Geometry check sheet. Reference: the model listing, model coordinates, mm. A direction names the side the tool comes from. Round coordinates to 2 decimals unless told otherwise and drop trailing zeros. Loops run counter-clockwise (first coordinate to the right, second up) from the corner with the lowest first, then second, coordinate; pieces in that order, holes last. Notation, with made-up numbers: M 75.5,10 L 111.5,10 A31 ccw 111.5,37 Z; hole C -9.5,-30 d5. An arc over 180 degrees is marked long. Use one line per item in the form item = value. Start each with the question number.
1. Go/stop test with flat-tipped pins: pin 1 (2 mm diameter, centred on y = 6, z = 18.5, fed in from +X); pin 2 (2 mm diameter, centred on x = 8, z = 0, fed in from -Y); pin 3 (2.5 mm diameter, centred on x = 8, y = -9, fed in from +Z); pin 4 (2.5 mm diameter, centred on x = 8.5, y = -8.5, fed in from -Z). Record where each tip stops, or that it passes through.
2. Cross-section at D-D (y = 5). Record the boundary of the cut face in (x, z), then the cut area to 3 significant figures.
3. Draft check along Y on faces 6 (the flat face through (10, -2.7, 2)), 7 (the flat face through (0, 25.2, 0)), 8 (the flat face through (-14, 21.752, 0)), 9 (the flat face through (8, -8, -2)). Enter one of: pulls with the +Y half, pulls with the -Y half, needs draft (parallel to the pull), parting line crosses it, or undercut.
4. Set-up check for faces 1 (the flat face through (-4, 1, 17)), 2 (the cylindrical face through (10.7, -0.6, 3.6)), 3 (the cylindrical face through (-13.72, 22.81, 4.19)), 4 (the cylindrical face through (-0.1, 1, 23.5)), 5 (the flat face through (8, -8, 2)): record each of +Z, -Z, +X, -X, +Y, -Y from which the full face is reachable in a straight line by a thin tool's end or side.
5. Cross-section at A-A (y = 1). Record the boundary of the cut face in (x, z).
6. Cross-section at B-B (x = 0). Record the boundary of the cut face in (y, z), then the cut area to 3 significant figures.
7. Cross-section at C-C (z = 10.5). Record the boundary of the cut face in (x, y), then the cut area to 3 significant figures.
8. Material ranges on line 1 (Z direction, x = 8, y = -8.05); line 2 (Y direction, x = -12.5, z = -3); line 3 (Y direction, x = 13, z = -2.5), recorded low to high.
```python
from build123d import *

# Parameters (mm, degrees)
HOLE_WIZARD_M3_1_D     = 2.5
HOLE_WIZARD_M3_1_DEPTH = 5
HOLE_WIZARD_M3_1_TIP   = 0.751075774
SKETCH_5_W             = 10.630358464
SKETCH_5_H             = 3.551561409
SKETCH_5_W_2           = 11.579063223
SKETCH_5_H_2           = 3.065046147
CUT_EXTRUDE_1_DEPTH    = 5
SKETCH_6_R             = 1.5
EXTRUDE_1_DEPTH        = 2
EXTRUDE_2_DEPTH        = 16


with BuildPart() as part:
    # 草图1 → 旋转1 (revolve)
    with BuildSketch(Plane.XY, mode=Mode.PRIVATE) as revolve_1_sk:
        Polygon((0, 0), (-16, 0), (-16, 12), (-13, 12), (-13, 14), (-12.25, 14), (-12.25, 25.2), (0, 25.2), align=None)
    revolve(revolve_1_sk.sketch.rotate(Axis((0, 0, 0), (0, 1, 0)), 270), axis=Axis((0, 0, 0), (0, 1, 0)))

    # 草图2 → 旋转2 (revolve)
    with BuildSketch(Plane.XY, mode=Mode.PRIVATE) as revolve_2_sk:
        Polygon((3.5, 0), (3.5, -1.25), (4, -1.25), (4, -2.7), (5.5, -2.7), (5.5, -10.2), (8, -10.2), (8, 0), align=None)
    revolve(revolve_2_sk.sketch.rotate(Axis((8, -10.2, 0), (0, 1, 0)), 270), axis=Axis((8, -10.2, 0), (0, 1, 0)))

    # M3 螺纹孔1
    with Locations(Plane(origin=(0, -10.2, 0), x_dir=(-1, 0, 0), z_dir=(0, -1, 0))):
        with Locations((-8, 0)):
            Hole(HOLE_WIZARD_M3_1_D / 2, depth=HOLE_WIZARD_M3_1_DEPTH)
            with Locations((0, 0, -(HOLE_WIZARD_M3_1_DEPTH + HOLE_WIZARD_M3_1_TIP / 2))):  # 118° drill point
                Cone(0, HOLE_WIZARD_M3_1_D / 2, HOLE_WIZARD_M3_1_TIP, mode=Mode.SUBTRACT)

    # 草图5 → 切除-拉伸1 (cut)
    with BuildSketch(Plane.XZ.offset(10.2)):
        with Locations((8.725419138, 3.775780705)):
            Rectangle(SKETCH_5_W, SKETCH_5_H)
        with Locations((9.759264069, -3.532523074)):
            Rectangle(SKETCH_5_W_2, SKETCH_5_H_2)
    extrude(amount=-CUT_EXTRUDE_1_DEPTH, mode=Mode.SUBTRACT)

    # 草图6 → 凸台-拉伸1 (add)
    with BuildSketch(Plane.XZ):
        with BuildLine():
            Line((-4, -19.5), (-4, 19.5))
            ThreePointArc((-4, 19.5), (0, 23.5), (4, 19.5))
            Line((4, 19.5), (4, -19.5))
            ThreePointArc((4, -19.5), (0, -23.5), (-4, -19.5))
        make_face()
        with Locations(Location((0, -19.5, 0), (0, 0, 270))):
            Circle(SKETCH_6_R, mode=Mode.SUBTRACT)
        with Locations(Location((0, 19.5, 0), (0, 0, 270))):
            Circle(SKETCH_6_R, mode=Mode.SUBTRACT)
    extrude(amount=-EXTRUDE_1_DEPTH)

    # 草图7 → 凸台-拉伸2 (add)
    with BuildSketch(Plane(origin=(0, 0, 0), x_dir=(0, 0, -1), z_dir=(1, 0, 0))):
        with BuildLine():
            Line((3.07585982, 21.752332949), (-3.109660478, 21.752332949))
            ThreePointArc((-3.109660478, 21.752332949), (-4.188603578, 22.83127605), (-3.109660478, 23.91021915))
            Line((-3.109660478, 23.91021915), (3.07585982, 23.91021915))
            ThreePointArc((3.07585982, 23.91021915), (4.154802921, 22.83127605), (3.07585982, 21.752332949))
        make_face()
    extrude(amount=-EXTRUDE_2_DEPTH)


solid = part.part
```
Reported:
q1.pin_1 = through
q1.pin_2 = -5.05
q1.pin_3 = 2
q1.pin_4 = -2
q2.outline = C 0,0 d32
q2.area = 804 mm²
q3.face_6 = pulls with the -Y half
q3.face_7 = pulls with the +Y half
q3.face_8 = undercut
q3.face_9 = needs draft
q4.face_1 = +Z, -X, +Y, -Y
q4.face_2 = -Y
q4.face_3 = +Z, -X
q4.face_4 = +Z, +Y, -Y
q4.face_5 = +Z, +X, -X, -Y
q5.outline = M -4,-19.5 A4 ccw 4,-19.5 L 4,-15.49 A16 ccw 4,15.49 L 4,19.5 A4 ccw -4,19.5 L -4,15.49 A16 ccw -4,-15.49 Z; hole C 0,-19.5 d3; hole C 0,19.5 d3
q6.outline = M 0,-23.5 L 2,-23.5 L 2,-21 L 0,-21 Z; M 0,-18 L 2,-18 L 2,-16 L 12,-16 L 12,-13 L 14,-13 L 14,-12.25 L 25.2,-12.25 L 25.2,12.25 L 14,12.25 L 14,13 L 12,13 L 12,16 L 2,16 L 2,18 L 0,18 Z; M 0,21 L 2,21 L 2,23.5 L 0,23.5 Z
q6.area = 728 mm²
q7.outline = M -12.07,0 L 12.07,0 L 12.07,12 L 7.66,12 L 7.66,14 L 6.31,14 L 6.31,25.2 L -6.31,25.2 L -6.31,14 L -7.66,14 L -7.66,12 L -12.07,12 Z
q7.area = 462 mm²
q8.line_1 = -2 to -1.25, 1.25 to 2
q8.line_2 = 0 to 14, 21.75 to 23.91
q8.line_3 = 0 to 12
